Autodesk Inventor part; units mm, degrees
ref_plane "YZ Plane" through (0, 0, 0) normal (1, 0, 0) x (0, 1, 0)
ref_plane "XZ Plane" through (0, 0, 0) normal (0, 1, 0) x (-1, 0, 0)
ref_plane "XY Plane" through (0, 0, 0) normal (0, 0, 1) x (1, 0, 0)
sketch "Sketch1" plane through (0, 0, 0) normal (0, 1, 0) x (-1, 0, 0)
  line L0 (0, 0) -> (25.4, 0)
  line L1 (25.4, 0) -> (25.4, 101.6)
  line L2 (25.4, 101.6) -> (0, 101.6)
  line L3 (0, 101.6) -> (0, 0)
  line L4 (12.7, 101.6) -> (12.7, 0) construction
  circle A0 centre (12.7, 12.7) radius 3.302
  circle A1 centre (12.7, 63.5) radius 3.302
  circle A2 centre (12.7, 88.9) radius 3.302
  line L5 (0, 0) -> (-25.4, 0)
  line L6 (-25.4, 0) -> (-25.4, 101.6)
  line L7 (-25.4, 101.6) -> (0, 101.6)
  dimension "d0" = 101.6
  dimension "d2" = 25.4
  dimension "d3" = 6.604
  dimension "d4" = 25.4
  dimension "d5" = 50.8
  dimension "d6" = 12.7
  dimension "d8" = 25.4
extrude "Plate1" add sketch "Sketch1" along normal blind 3.175
sketch "Sketch2" plane through (22.225, 0, 0) normal (1, 0, 0) x (0, 1, 0)
  line L0 (0, 101.6) -> (0, 0)
  line L1 (0, 0) -> (152.4, 0)
  line L2 (152.4, 0) -> (152.4, 101.6)
  line L3 (152.4, 101.6) -> (0, 101.6)
edge flange "Flange1" height 152.4 angle 90 thickness 3.175 bend radius 1.27 thickness toward (1, 0, 0) relief straight relief width 3.175 relief depth 1.5875 edges at (25.4, 3.175, 50.8) wall of the first edge with corners at (22.225, 0, 101.6) (22.225, 0, 0) (22.225, 152.4, 0) (22.225, 152.4, 101.6)
bend "Bend1"
corner "Corner1"
sketch "Sketch3" plane through (25.4, 152.4, 101.6) normal (1, 0, 0) x (0, 0, -1)
  line L0 (0, -147.955) -> (101.6, -147.955)
  line L1 (101.6, 0) -> (101.6, -147.955)
  line L2 (0, 0) -> (101.6, 0)
  line L3 (0, -147.955) -> (0, 0)
  line L4 (12.7, -74.295) -> (27.94, -74.295) construction
  line L5 (27.94, -74.295) -> (27.94, -127) construction
  line L6 (27.94, -127) -> (12.7, -127) construction
  line L7 (12.7, -127) -> (12.7, -74.295) construction
  circle A0 centre (12.7, -74.295) radius 2.2225
  circle A1 centre (27.94, -74.295) radius 2.2225
  circle A2 centre (27.94, -127) radius 2.2225
  circle A3 centre (12.7, -127) radius 2.2225
  line L8 (101.6, -152.4) -> (0, -152.4) construction
  circle A4 centre (44.3804, -106.4123) radius 2.2225
  line L9 (44.3804, -106.4123) -> (82.4804, -106.4123) construction
  circle A5 centre (82.4804, -106.4123) radius 2.2225
  dimension "d19" = 52.705
  dimension "d21" = 15.24
  dimension "d22" = 4.445
  dimension "d23" = 25.4
  dimension "d24" = 12.7
  dimension "d25" = 38.1
  dimension "d26" = 4.445
equation "\"d9\" = BendReliefWidth"
equation "\"d10\" = BendReliefDepth"
equation "\"d11\" = MinimumRemnant"
equation "\"d12\" = BendRadius"
equation "\"d16\" = CornerReliefSize"
equation "\"d17\" = GapSize"
equation "\"d18\" = JacobiRadiusSize"
equation "\"BendRadius\" = Thickness"
equation "\"BendReliefWidth\" = Thickness"
equation "\"BendReliefDepth\" = 0.5 * Thickness"
equation "\"CornerReliefSize\" = 4 * Thickness"
equation "\"MinimumRemnant\" = 2 * Thickness"
equation "\"TransitionRadius\" = BendRadius"
equation "\"JacobiRadiusSize\" = Thickness"
equation "\"GapSize\" = Thickness"
equation "\"d7\" = BendRadius"
properties part number "Pneumatic Mount Bracket" material "Aluminum 6061"
Can you work these out from the model? Positions are in its coordinate system, mm. A direction names the side the tool comes from. Coordinates: 2 decimals unless noted, no trailing zeros. Write each loop counter-clockwise with the first axis right and the second up, starting at its lowest first coordinate (ties: lowest second). Pieces come first, ordered by that corner, then holes.
Q1. Please list where these lines run through material, in increasing order: L1, parallel to Z at x = -12.7, y = 1.1; L2, parallel to Z at x = -12, y = 1; L3, parallel to Y at x = -4, z = 31.5 (3 decimals).
Results found:
L1: z = 0 to 9.4, 16 to 60.2, 66.8 to 85.6, 92.2 to 101.6
L2: z = 0 to 9.47, 15.93 to 60.27, 66.73 to 85.67, 92.13 to 101.6
L3: y = 0 to 3.175
Q2. Imagine slicing it at B-B, the plane z = 88.9. List the corners of the cut face in (x, y) for me (3 decimals).
Results found:
outline: (-25.4, 0) - (-16.002, 0) - (-16.002, 3.175) - (-25.4, 3.175) - close; (-9.398, 0) - (20.955, 0) arc R4.445 ccw to (25.4, 4.445) - (25.4, 152.4) - (22.225, 152.4) - (22.225, 4.445) arc R1.27 cw to (20.955, 3.175) - (-9.398, 3.175) - close
Q3. Imagine slicing it at A-A, the plane x = -12.7. List the corners of the cut face in (y, z) for me (3 decimals).
Results found:
outline: (0, 0) - (3.175, 0) - (3.175, 9.398) - (0, 9.398) - close; (0, 16.002) - (3.175, 16.002) - (3.175, 60.198) - (0, 60.198) - close; (0, 66.802) - (3.175, 66.802) - (3.175, 85.598) - (0, 85.598) - close; (0, 92.202) - (3.175, 92.202) - (3.175, 101.6) - (0, 101.6) - close
Q4. Imagine slicing it at D-D, the plane y = 129. List the corners of the cut face in (x, z) for me (3 decimals), plus the area to 3 significant figures.
Results found:
outline: (22.225, 0) - (25.4, 0) - (25.4, 101.6) - (22.225, 101.6) - close
area: 323 mm2
Q5. If we mould it in two halves opening along Z, with no side actions, what happens to faces 3 (the face through (-11.984, 1.565, 15.923)), 4 (the face through (23, 77, 101.6)), 5 (the face through (-2, 3.175, 52))? For each: +Z half, -Z half, draft (parallel to the pull), parting line (faces both ways), or undercut.
Results found:
face 3: undercut
face 4: +Z half
face 5: draft
Q6. Which directions (+Z, -Z, +X, -X, +Y, -Y) give clear straight access to the entire face, cutting with the end or side of a thin tool? Please do faces 1 (the face through (22.225, 77, 50)), 2 (the face through (23, 77, 0)).
Results found:
face 1: +Z, -Z, -X, +Y
face 2: -Z, +X, -X, +Y, -Y
Q7. Imagine slicing it at C-C, the plane z = 39. List the corners of the cut face in (x, y) for me (3 decimals).
Results found:
outline: (-25.4, 0) - (20.955, 0) arc R4.445 ccw to (25.4, 4.445) - (25.4, 152.4) - (22.225, 152.4) - (22.225, 4.445) arc R1.27 cw to (20.955, 3.175) - (-25.4, 3.175) - close
Q8. For P1, Ø3, axis at y = 87.5, z = 42, coming from the -X side (3 decimals); P2, Ø12, axis at x = -6, z = 45.5, coming from the +Y side (3 decimals); P3, Ø5.5, axis at x = -12.7, z = 88.9, coming from the -Y side, each with a flat end and sliding along its axis, tell me the tip position at first contact or that it passes through.
Results found:
P1: stops at x = 22.225
P2: stops at y = 3.175
P3: passes through
